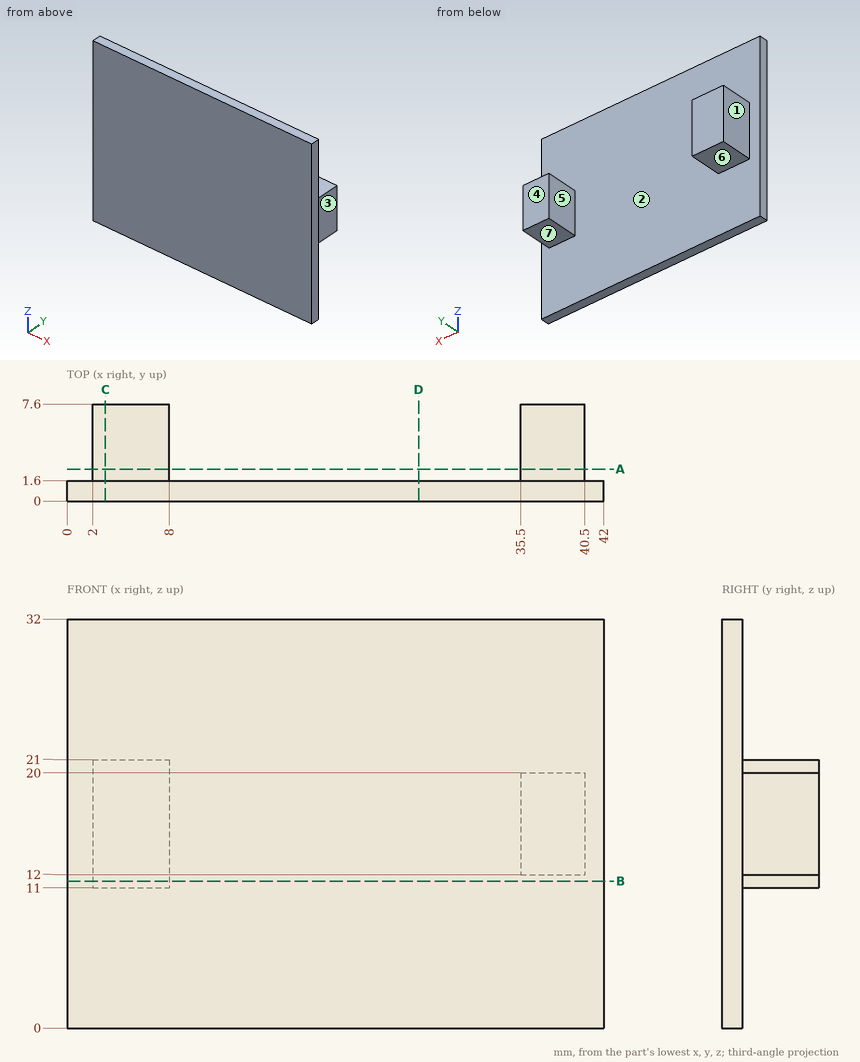
Geometry check sheet. Reference: drawing and pictorial views, mm from the part's lowest x, y, z. A direction names the side the tool comes from. Round coordinates to 2 decimals unless told otherwise and drop trailing zeros. Loops run counter-clockwise (first coordinate to the right, second up) from the corner with the lowest first, then second, coordinate; pieces in that order, holes last.
1. Sectioned sample at D-D on x = 27.5. Record the boundary of the cut face in (y, z).
2. Mould release check, pull along X, two halves, no side actions. Record for the marked faces 1, 2, 3 and 4: released by +X, released by -X, zero draft, split by the parting line, or undercut.
3. Sectioned sample at C-C on x = 3. Record the boundary of the cut face in (y, z).
4. Scan lines: probe 1 along X at (y, z) = (2.75, 14); probe 2 along Y at (x, z) = (19, 25.5); probe 3 along Z at (x, y) = (4, 6). Record each from-to range of solid material in increasing order.
5. Sectioned sample at A-A on y = 2.5. Record the boundary of the cut face in (x, z).
6. Gauge pin test, flat ends, axial feed: pin 1 Ø6 at (x, z) = (27, 26.5) entering from +Y; pin 2 Ø1.5 at (x, y) = (37, 5.5) entering from +Z; pin 3 Ø3 at (y, z) = (5, 18) entering from +X. Record the tip position at first contact, or that the pin passes through.
7. Set-up check for the marked faces 5, 6 and 7: record each of +Z, -Z, +X, -X, +Y, -Y from which the full face is reachable in a straight line by a thin tool's end or side.
8. Sectioned sample at B-B on z = 11.5. Record the boundary of the cut face in (x, y).
Recorded:
1. outline: (0, 0) - (1.6, 0) - (1.6, 32) - (0, 32) - close
2. face 1: released by -X
2. face 2: undercut
2. face 3: released by +X
2. face 4: zero draft
3. outline: (0, 0) - (1.6, 0) - (1.6, 11) - (7.6, 11) - (7.6, 21) - (1.6, 21) - (1.6, 32) - (0, 32) - close
4. probe 1: x = 2 to 8, 35.5 to 40.5
4. probe 2: y = 0 to 1.6
4. probe 3: z = 11 to 21
5. outline: (2, 11) - (8, 11) - (8, 21) - (2, 21) - close; (35.5, 12) - (40.5, 12) - (40.5, 20) - (35.5, 20) - close
6. pin 1: stops at y = 1.6
6. pin 2: stops at z = 20
6. pin 3: stops at x = 40.5
7. face 5: +Z, -Z, +Y
7. face 6: -Z, +X, -X, +Y
7. face 7: -Z, +X, +Y
8. outline: (0, 0) - (42, 0) - (42, 1.6) - (8, 1.6) - (8, 7.6) - (2, 7.6) - (2, 1.6) - (0, 1.6) - close
